Verification items for the finished model (mm, model axes). Face numbers are marked on the shaded views. A direction names the side the tool comes from. Give positions to 0.01 mm unless a question says otherwise; leave off trailing zeros. Write each loop counter-clockwise with the first axis right and the second up, starting at its lowest first coordinate (ties: lowest second). Pieces come first, ordered by that corner, then holes. Notation, with made-up numbers: (61, 39) -> (70, 39) arc R26 ccw to (70, 56) -> close; hole circle Ø7 at (39.5, 37). An arc over 180 degrees is marked (long way). Answer as CSV lines item,"result". Start each with the question number.
1) Tool access check on the marked faces 1, 2, 3, 4 and 5. Record the directions out of +Z, -Z, +X, -X, +Y, -Y that give a thin tool (end or side, any length) a straight path to the whole face; none if there is none.
2) Sectioned sample at A-A on x = 5. Record the cut outline in (y, z).
3) Material ranges on L1, parallel to X at y = 9, z = 7.75; L2, parallel to Y at x = 17.5, z = 2.5; L3, parallel to Z at x = 31.5, y = 3.5, recorded low to high.
4) Sectioned sample at B-B on z = 4.5. Record the cut outline in (x, y), and give its area (3 significant figures).
5) Sectioned sample at D-D on z = 1. Record the cut outline in (x, y), and give its area (3 significant figures).
6) Gauge pin test, flat ends, axial feed: pin 1 Ø3 at (x, y) = (53, 3.5) entering from +Z; pin 2 Ø5 at (y, z) = (2.5, 5) entering from +X; pin 3 Ø3 at (x, y) = (6, 6) entering from +Z; pin 4 Ø3 at (x, y) = (65, 5) entering from -Z. Record the tip position at first contact, or that the pin passes through.
7) Sectioned sample at C-C on y = 5. Record the cut outline in (x, z).
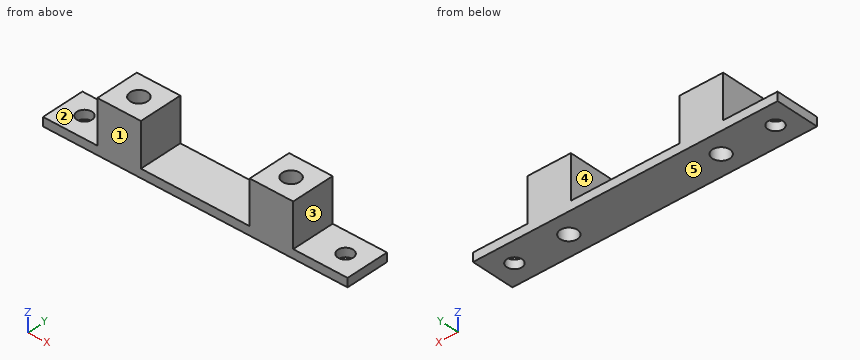
```python
from build123d import *

# Parameters (mm, degrees)
ESQUISSE2_W             = 70
ESQUISSE2_H             = 10
BOSS_EXTRU_1_DEPTH      = 2
ESQUISSE3_W             = 10
ESQUISSE3_H             = 10
BOSS_EXTRU_2_DEPTH      = 10
ESQUISSE4_R             = 2
ESQUISSE4_R_2           = 1.75
ENL_V_MAT_EXTRU_1_DEPTH = 20


with BuildPart() as part:
    # Esquisse2 → Boss.-Extru.1 (new body)
    with BuildSketch(Plane.XY):
        with Locations((35, 5)):
            Rectangle(ESQUISSE2_W, ESQUISSE2_H)
    extrude(amount=BOSS_EXTRU_1_DEPTH)

    # Esquisse3 → Boss.-Extru.2 (add)
    with BuildSketch(Plane.XY.offset(2)):
        with Locations((17.5, 5)):
            Rectangle(ESQUISSE3_W, ESQUISSE3_H)
        with Locations((52.5, 5)):
            Rectangle(ESQUISSE3_W, ESQUISSE3_H)
    extrude(amount=BOSS_EXTRU_2_DEPTH)

    # Esquisse4 → Enlèv. mat.-Extru.1 (cut)
    with BuildSketch(Plane.XY.offset(12)):
        with Locations((52.5, 5)):
            Circle(ESQUISSE4_R)
        with Locations((17.5, 5)):
            Circle(ESQUISSE4_R)
        with Locations(Location((5, 5, 0), (0, 0, 180))):
            Circle(ESQUISSE4_R_2)
        with Locations(Location((65, 5, 0), (0, 0, 180))):
            Circle(ESQUISSE4_R_2)
    extrude(amount=-ENL_V_MAT_EXTRU_1_DEPTH, mode=Mode.SUBTRACT)


solid = part.part
```
Ans:
1,face 1,"+Z, -Z, +X, -X, -Y"
1,face 2,"+Z, -X, +Y, -Y"
1,face 3,"+Z, +X, +Y, -Y"
1,face 4,"+Z, +Y, -Y"
1,face 5,"-Z, +X, -X, +Y, -Y"
2,outline,"(0, 0) -> (3.25, 0) -> (3.25, 2) -> (0, 2) -> close; (6.75, 0) -> (10, 0) -> (10, 2) -> (6.75, 2) -> close"
3,L1,"x = 12.5 to 22.5, 47.5 to 57.5"
3,L2,"y = 0 to 3, 7 to 10"
3,L3,"z = 0 to 2"
4,outline,"(12.5, 0) -> (22.5, 0) -> (22.5, 10) -> (12.5, 10) -> close; (47.5, 0) -> (57.5, 0) -> (57.5, 10) -> (47.5, 10) -> close; hole circle Ø4 at (17.5, 5); hole circle Ø4 at (52.5, 5)"
4,area,"175 mm²"
5,outline,"(0, 0) -> (70, 0) -> (70, 10) -> (0, 10) -> close; hole circle Ø3.5 at (5, 5); hole circle Ø4 at (17.5, 5); hole circle Ø4 at (52.5, 5); hole circle Ø3.5 at (65, 5)"
5,area,"656 mm²"
6,pin 1,"stops at z = 12"
6,pin 2,"stops at x = 57.5"
6,pin 3,"stops at z = 2"
6,pin 4,"passes through"
7,outline,"(0, 0) -> (3.25, 0) -> (3.25, 2) -> (0, 2) -> close; (6.75, 0) -> (15.5, 0) -> (15.5, 12) -> (12.5, 12) -> (12.5, 2) -> (6.75, 2) -> close; (19.5, 0) -> (50.5, 0) -> (50.5, 12) -> (47.5, 12) -> (47.5, 2) -> (22.5, 2) -> (22.5, 12) -> (19.5, 12) -> close; (54.5, 0) -> (63.25, 0) -> (63.25, 2) -> (57.5, 2) -> (57.5, 12) -> (54.5, 12) -> close; (66.75, 0) -> (70, 0) -> (70, 2) -> (66.75, 2) -> close"
